Read the model definition and answer for the solid it produces. Units are mm, in the model's axes. Face numbers are marked on the shaded views. A direction names the side the tool comes from. Coordinates: 2 decimals unless noted, no trailing zeros. Loops run counter-clockwise (first coordinate to the right, second up) from the corner with the lowest first, then second, coordinate; pieces in that order, holes last.
Q1. Which of the six approach directions +Z, -Z, +X, -X, +Y, -Y give full straight-line access (tool end or side, diameter ignored) to the marked faces 5, 6 and 7?
Q2. Section C-C (x = 3.5) is taken. Give the vertices of the cut face in (y, z).
Q3. Section D-D (y = 20.5) is taken. Give the vertices of the cut face in (x, z).
Q4. Straight lines are drawn through the part: line 1 (X direction, y = 33.5, z = -13.25); line 2 (X direction, y = 33, z = 11); line 3 (Y direction, x = 3.5, z = 12.15). For each, find the intervals that lie inside material, in ascending order.
Q5. The mould has two halves that part along Y. Classify the marked faces 1, 2, 3 and 4: pulls with the +Y half, pulls with the -Y half, needs draft (parallel to the pull), parting line crosses it, or undercut.
Q6. Section A-A (z = -5.5) is taken. Give the vertices of the cut face in (x, y).
Q7. Flat-ended cylindrical pins translate along their axes: P1, Ø0.8, axis at x = 3, y = 33.5, coming from the +Z side; P2, Ø2, axis at x = 66.5, y = 3.5, coming from the -Z side. Find the tip coordinate at first contact, or state that the pin passes through.
Q8. Section B-B (y = 31) is taken. Give the vertices of the cut face in (x, z), then the cut area to 3 significant figures.
from build123d import *

# Parameters (mm, degrees)
SKETCH1_W                = 70
SKETCH1_H                = 37
BOSS_EXTRUDE1_DEPTH      = 10
BOSS_EXTRUDE4_DEPTH      = 14
BOSS_EXTRUDE4_DEPTH_BACK = 30
SKETCH2_W                = 7
SKETCH2_H                = 7
SKETCH2_R                = 1.25


with BuildPart() as part:
    # Sketch1 → Boss-Extrude1 (new body)
    with BuildSketch(Plane.XY):
        with Locations((35, 18.5)):
            Rectangle(SKETCH1_W, SKETCH1_H)
    extrude(amount=BOSS_EXTRUDE1_DEPTH)

    # Sketch2 → Boss-Extrude4 (add, two sides: drawn at the far end of the back side and taken through both)
    # profile 1 of 4: a face of its own
    with BuildSketch(Plane.XY.offset(-BOSS_EXTRUDE4_DEPTH_BACK)):
        with Locations((3.5, 33.5)):
            Rectangle(SKETCH2_W, SKETCH2_H)
        with Locations((3.5, 33.5)):
            Circle(SKETCH2_R, mode=Mode.SUBTRACT)
    # profile 2 of 4: a face of its own
    with BuildSketch(Plane.XY.offset(-BOSS_EXTRUDE4_DEPTH_BACK)):
        with Locations((66.5, 33.5)):
            Rectangle(SKETCH2_W, SKETCH2_H)
        with Locations((66.5, 33.5)):
            Circle(SKETCH2_R, mode=Mode.SUBTRACT)
    # profile 3 of 4: a face of its own
    with BuildSketch(Plane.XY.offset(-BOSS_EXTRUDE4_DEPTH_BACK)):
        with Locations((66.5, 3.5)):
            Rectangle(SKETCH2_W, SKETCH2_H)
        with Locations((66.5, 3.5)):
            Circle(SKETCH2_R, mode=Mode.SUBTRACT)
    # profile 4 of 4: a face of its own
    with BuildSketch(Plane.XY.offset(-BOSS_EXTRUDE4_DEPTH_BACK)):
        with Locations((3.5, 3.5)):
            Rectangle(SKETCH2_W, SKETCH2_H)
        with Locations((3.5, 3.5)):
            Circle(SKETCH2_R, mode=Mode.SUBTRACT)
    extrude(amount=BOSS_EXTRUDE4_DEPTH + BOSS_EXTRUDE4_DEPTH_BACK)


solid = part.part
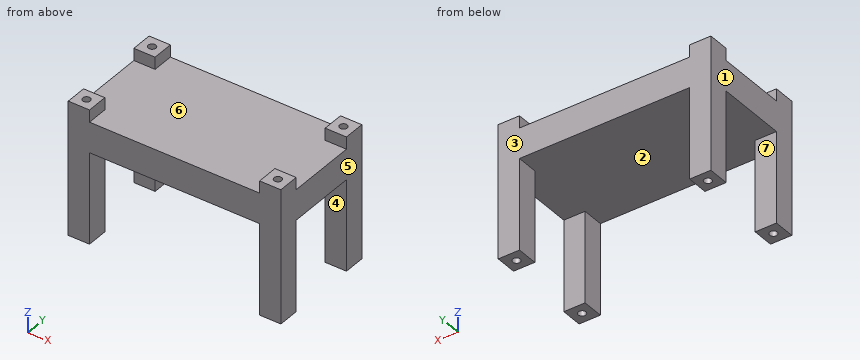
Numbers:
1. face 5: +Z, -Z, +X, +Y, -Y
1. face 6: +Z
1. face 7: -Z, +X, -X
2. outline: (0, -30) - (2.25, -30) - (2.25, 0) - (4.75, 0) - (4.75, -30) - (7, -30) - (7, 0) - (30, 0) - (30, -30) - (32.25, -30) - (32.25, 0) - (34.75, 0) - (34.75, -30) - (37, -30) - (37, 14) - (34.75, 14) - (34.75, 10) - (32.25, 10) - (32.25, 14) - (30, 14) - (30, 10) - (7, 10) - (7, 14) - (4.75, 14) - (4.75, 10) - (2.25, 10) - (2.25, 14) - (0, 14) - close
3. outline: (0, 0) - (70, 0) - (70, 10) - (0, 10) - close
4. line 1: x = 0 to 2.25, 4.75 to 7, 63 to 65.25, 67.75 to 70
4. line 2: x = 0 to 2.35, 4.65 to 7, 63 to 65.35, 67.65 to 70
4. line 3: y = 0 to 2.25, 4.75 to 7, 30 to 32.25, 34.75 to 37
5. face 1: needs draft
5. face 2: undercut
5. face 3: pulls with the +Y half
5. face 4: undercut
6. outline: (0, 0) - (7, 0) - (7, 7) - (0, 7) - close; (0, 30) - (7, 30) - (7, 37) - (0, 37) - close; (63, 0) - (70, 0) - (70, 7) - (63, 7) - close; (63, 30) - (70, 30) - (70, 37) - (63, 37) - close; hole circle Ø2.5 at (3.5, 3.5); hole circle Ø2.5 at (3.5, 33.5); hole circle Ø2.5 at (66.5, 3.5); hole circle Ø2.5 at (66.5, 33.5)
7. P1: stops at z = 10
7. P2: stops at z = 0
8. outline: (0, -30) - (7, -30) - (7, 0) - (63, 0) - (63, -30) - (70, -30) - (70, 14) - (63, 14) - (63, 10) - (7, 10) - (7, 14) - (0, 14) - close
8. area: 1,180 mm2
